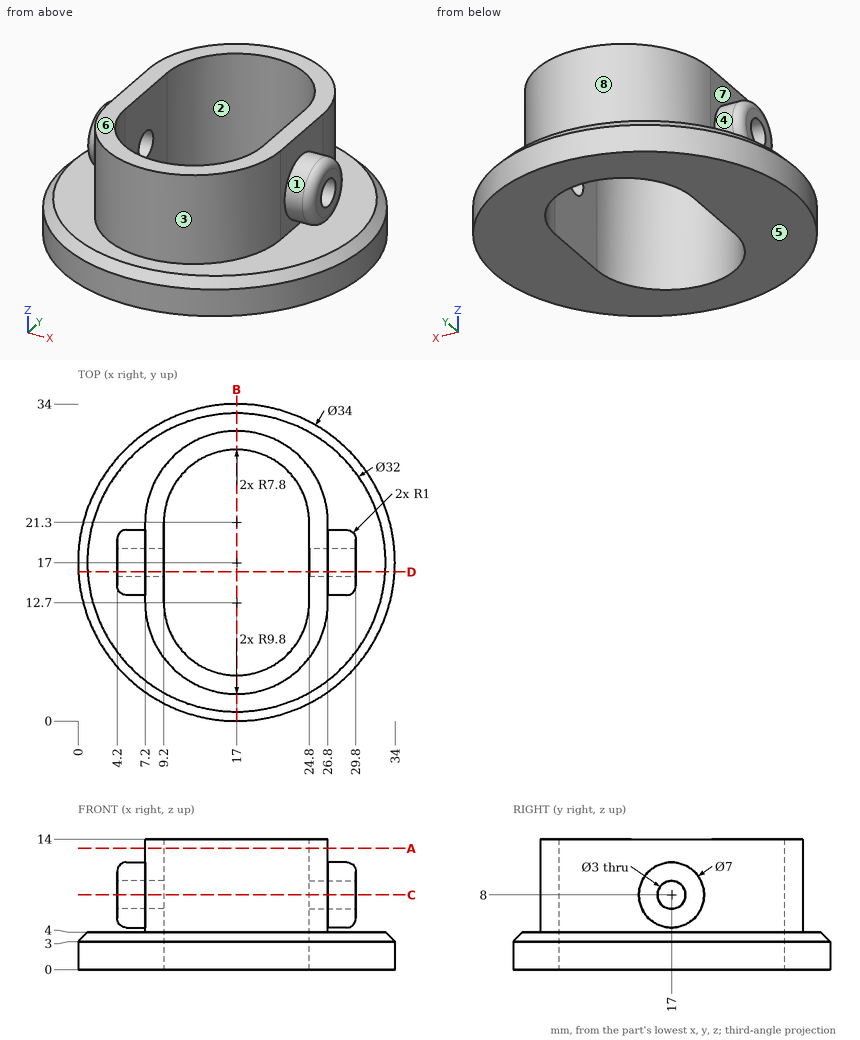
Here's the drawing with two shaded views (mm, measured from the low corner). I have some questions. A direction names the side the tool comes from. Give positions to 0.01 mm unless a question says otherwise; leave off trailing zeros. Loops run counter-clockwise (first coordinate to the right, second up) from the corner with the lowest first, then second, coordinate; pieces in that order, holes last. Notation, with made-up numbers: (19.5, 71) -> (38.5, 71) arc R6 ccw to (38.5, 77) -> close; hole circle Ø8 at (-26.5, 68). An arc over 180 degrees is marked (long way). Use one line per item in the form item = value.
1) I need wall thicknesses on line 1 along Z through (x, y) = (28, 17); line 2 along X through (y, z) = (21.5, 12.75); line 3 along X through (y, z) = (17, 5.75). Which ranges of each line are inside material? Lowest first, please.
Answers:
line_1 = 0 to 4, 4.5 to 6.5, 9.5 to 11.5
line_2 = 7.2 to 9.2, 24.8 to 26.8
line_3 = 4.2 to 9.2, 24.8 to 29.8
2) Will these pins go through, and if not, where does the flat tip stop? pin 1 (1 mm diameter, centred on x = 6, y = 28, fed in from +Z); pin 2 (4 mm diameter, centred on x = 7.5, z = 10.5, fed in from +Y); pin 3 (1 mm diameter, centred on x = 10.5, y = 22.5, fed in from -Z); pin 4 (3 mm diameter, centred on x = 24, y = 13.5, fed in from -Z).
Answers:
pin_1 = 4
pin_2 = 27.61
pin_3 = through
pin_4 = 0
3) For the marked faces 1, 2, 3 and 4, which set-ups out of +Z, -Z, +X, -X, +Y, -Y let a thin tool reach every point of the face, with its end or its side?
Answers:
face_1 = +X
face_2 = +Z, -Z
face_3 = +Z, -Y
face_4 = -X
4) If we section it at B-B (x = 17): Please give me the cut outline in (y, z).
Answers:
outline = (0, 0) -> (4.9, 0) -> (4.9, 14) -> (2.9, 14) -> (2.9, 4) -> (1, 4) -> (0, 3) -> close; (29.1, 0) -> (34, 0) -> (34, 3) -> (33, 4) -> (31.1, 4) -> (31.1, 14) -> (29.1, 14) -> close
5) We'd pull the mould along Z, two halves only. Please class the marked faces 5, 6, 7 and 8: released by +Z, released by -Z, zero draft, split by the parting line, or undercut.
Answers:
face_5 = released by -Z
face_6 = released by +Z
face_7 = undercut
face_8 = zero draft
6) If we section it at A-A (z = 13): Please give me the cut outline in (x, y).
Answers:
outline = (7.2, 12.7) arc R9.8 ccw to (26.8, 12.7) -> (26.8, 21.3) arc R9.8 ccw to (7.2, 21.3) -> close; hole (9.2, 12.7) arc R7.8 ccw to (24.8, 12.7) -> (24.8, 21.3) arc R7.8 ccw to (9.2, 21.3) -> close
7) If we section it at C-C (z = 8): Please give me the cut outline in (x, y), plus the area to 3 significant figures.
Answers:
outline = (4.2, 14.5) arc R1 ccw to (5.2, 13.5) -> (7.2, 13.5) -> (7.2, 12.7) arc R9.8 ccw to (26.8, 12.7) -> (26.8, 13.5) -> (28.8, 13.5) arc R1 ccw to (29.8, 14.5) -> (29.8, 15.5) -> (24.8, 15.5) -> (24.8, 12.7) arc R7.8 cw to (9.2, 12.7) -> (9.2, 15.5) -> (4.2, 15.5) -> close; (4.2, 18.5) -> (9.2, 18.5) -> (9.2, 21.3) arc R7.8 cw to (24.8, 21.3) -> (24.8, 18.5) -> (29.8, 18.5) -> (29.8, 19.5) arc R1 ccw to (28.8, 20.5) -> (26.8, 20.5) -> (26.8, 21.3) arc R9.8 ccw to (7.2, 21.3) -> (7.2, 20.5) -> (5.2, 20.5) arc R1 ccw to (4.2, 19.5) -> close
area = 156 mm²
8) If we section it at D-D (y = 16): Count the separate pieces of the cut face and the enclosed holes in it, plus the area to 3 significant figures.
Answers:
separate_pieces = 4
enclosed_holes = 0
area = 129 mm²
